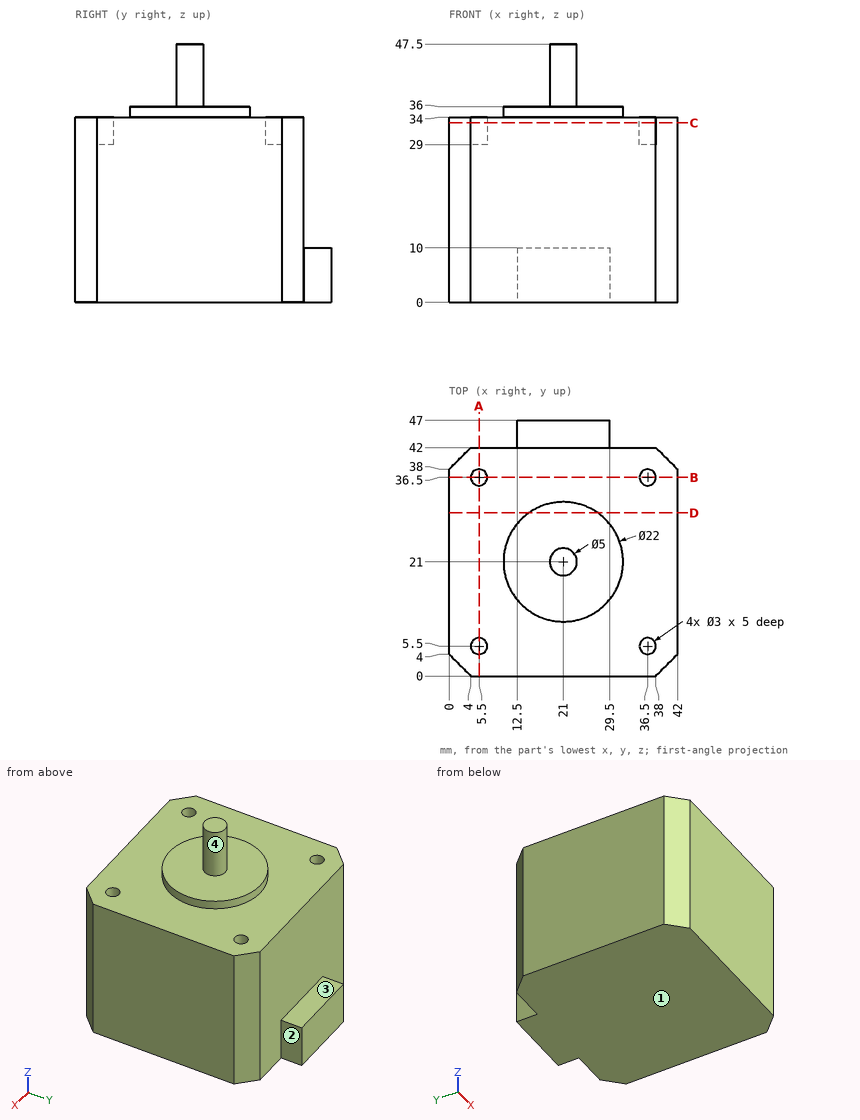
Study the drawing (mm; zero at the part's minimum x, y, z) and answer. A direction names the side the tool comes from. Coordinates: 2 decimals unless noted, no trailing zeros. Loops run counter-clockwise (first coordinate to the right, second up) from the corner with the lowest first, then second, coordinate; pieces in that order, holes last. Notation, with made-up numbers: (84, 41) -> (88, 41) arc R27 ccw to (88, 75) -> close; hole circle Ø8 at (66, 48). An arc over 180 degrees is marked (long way). Answer in a Markdown table with one row per item. Add a question column.
1. Consider line 1 (Y direction, x = 36.5, z = 32.85); line 2 (Z direction, x = 9, y = 28.5); line 3 (Y direction, x = 30.5, z = 30.5). Determine where each line is inside the solid, lowest interval first. Write a range as [from, to].
2. Flat-ended cylindrical pins translate along their axes: P1, Ø1.5, axis at x = 37, y = 6, coming from the +Z side; P2, Ø2.5, axis at x = 37, y = 36.5, coming from the +Z side; P3, Ø2.5, axis at y = 45, z = 5.5, coming from the -X side. Find the tip coordinate at first contact, or state that the pin passes through.
3. For the marked faces 1, 2, 3 and 4, determine the directions among +Z, -Z, +X, -X, +Y, -Y from which every point of the face is accessible in a straight line to the end or side of a thin tool.
4. The part is cut by section A-A, the plane x = 5.5. Write down the section's boundary in (y, z), then the cut area to 3 significant figures.
5. The part is cut by section C-C, the plane z = 33. Write down the section's boundary in (x, y), then the cut area to 3 significant figures.
6. The part is cut by section D-D, the plane y = 30. Write down the section's boundary in (x, z), then the cut area to 3 significant figures.
Answer below:
| question | item | result |
|---|---|---|
| 1 | line 1 | [0, 4], [7, 35], [38, 42] |
| 1 | line 2 | [0, 34] |
| 1 | line 3 | [0, 42] |
| 2 | P1 | z = 29 |
| 2 | P2 | z = 34 |
| 2 | P3 | x = 12.5 |
| 3 | face 1 | -Z, +X, -X, +Y, -Y |
| 3 | face 2 | +Z, -Z, +X, +Y |
| 3 | face 3 | +Z, +X, -X, +Y |
| 3 | face 4 | +Z |
| 4 | outline | (0, 0) -> (42, 0) -> (42, 34) -> (38, 34) -> (38, 29) -> (35, 29) -> (35, 34) -> (7, 34) -> (7, 29) -> (4, 29) -> (4, 34) -> (0, 34) -> close |
| 4 | area | 1,400 mm2 |
| 5 | outline | (0, 4) -> (4, 0) -> (38, 0) -> (42, 4) -> (42, 38) -> (38, 42) -> (4, 42) -> (0, 38) -> close; hole circle Ø3 at (5.5, 5.5); hole circle Ø3 at (5.5, 36.5); hole circle Ø3 at (36.5, 5.5); hole circle Ø3 at (36.5, 36.5) |
| 5 | area | 1,700 mm2 |
| 6 | outline | (0, 0) -> (42, 0) -> (42, 34) -> (27.32, 34) -> (27.32, 36) -> (14.68, 36) -> (14.68, 34) -> (0, 34) -> close |
| 6 | area | 1,450 mm2 |
